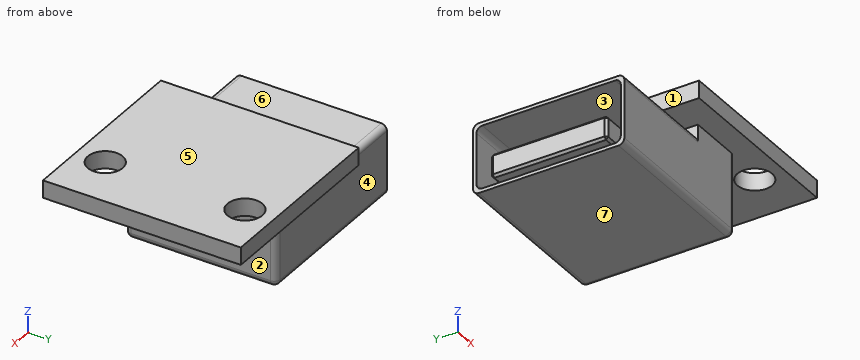
from build123d import *

# Parameters (mm, degrees)
SKETCH1_W           = 16
SKETCH1_H           = 17
BOSS_EXTRUDE1_DEPTH = 1.5
BOSS_EXTRUDE2_DEPTH = 6.5
SKETCH3_W           = 5.4
SKETCH3_H           = 12.4
SKETCH3_W_2         = 2
SKETCH3_H_2         = 10
CUT_EXTRUDE1_DEPTH  = 10
FILLET1_R           = 0.5
FILLET2_R           = 0.5
CHAMFER1_SIZE       = 0.2
SKETCH4_R           = 1.5
CUT_EXTRUDE2_DEPTH  = 10


with BuildPart() as part:
    # Sketch1 → Boss-Extrude1 (new body)
    with BuildSketch(Plane.XY):
        Rectangle(SKETCH1_W, SKETCH1_H)
    extrude(amount=BOSS_EXTRUDE1_DEPTH)

    # Sketch2 → Boss-Extrude2 (add, symmetric)
    with BuildSketch(Plane(origin=(0, 0, 0), x_dir=(1, 0, 0), z_dir=(0, 1, 0))):
        Polygon((-5, 0), (-5, 1), (-15, 1), (-15, 7), (0, 7), (0, 0), align=None)
    extrude(amount=BOSS_EXTRUDE2_DEPTH, both=True)

    # Sketch3 → Cut-Extrude1 (cut)
    with BuildSketch(Plane.ZY.offset(15)):
        with Locations((-4, 0)):
            Rectangle(SKETCH3_W, SKETCH3_H)
        with Locations((-5, 0)):
            Rectangle(SKETCH3_W_2, SKETCH3_H_2, mode=Mode.SUBTRACT)
    extrude(amount=-CUT_EXTRUDE1_DEPTH, mode=Mode.SUBTRACT)

    # Fillet1
    fillet1_edges = [part.edges().sort_by_distance(p)[0] for p in [
        (-7.5, -6.5, -7),
        (-10, -6.5, -1),
        (-7.5, 6.5, -7),
        (-10, 6.5, -1),
        (-10, 6.2, -6.7),
        (-10, 6.2, -1.3),
        (-10, -6.2, -1.3),
        (-10, -6.2, -6.7),
    ]]
    fillet(fillet1_edges, radius=FILLET1_R)

    # Fillet2
    fillet2_edges = [part.edges().sort_by_distance(p)[0] for p in [
        (0, -6.5, -3.25),
        (0, 6.5, -3.25),
        (0, 0, -7),
        (0, 6.353553391, -6.853553391),
        (0, -6.353553391, -6.853553391),
    ]]
    fillet(fillet2_edges, radius=FILLET2_R)

    # Chamfer1
    chamfer1_edges = [part.edges().sort_by_distance(p)[0] for p in [
        (-15, 0, -4),
        (-10, -5, -4),
        (-15, -5, -5),
        (-10, -5, -6),
        (-15, 0, -6),
        (-10, 5, -6),
        (-15, 5, -5),
        (-10, 5, -4),
    ]]
    chamfer(chamfer1_edges, length=CHAMFER1_SIZE)

    # Sketch4 → Cut-Extrude2 (cut)
    with BuildSketch(Plane(origin=(0, 0, 0), x_dir=(-1, 0, 0), z_dir=(0, 0, -1))):
        with Locations((-3.5, 6)):
            Circle(SKETCH4_R)
        with Locations((-3.5, -6)):
            Circle(SKETCH4_R)
    extrude(amount=-CUT_EXTRUDE2_DEPTH, mode=Mode.SUBTRACT)


solid = part.part
The listing builds one solid part. Answer for the finished solid, in the listing's coordinates (mm). Face numbers are marked on the shaded views. A direction names the side the tool comes from. Coordinates: 2 decimals unless noted, no trailing zeros. Write each loop counter-clockwise with the first axis right and the second up, starting at its lowest first coordinate (ties: lowest second). Pieces come first, ordered by that corner, then holes. Notation, with made-up numbers: (-40, 12) - (-19, 12) arc R21 cw to (-19, 22) - close; hole circle Ø10 at (58, 23.25). An arc over 180 degrees is marked (long way). Put each result on its own line as item: value.
1. Determine the mould class of the marked faces 4, 5, 6 and 7 for opening direction Z: pulls with the +Z half, pulls with the -Z half, needs draft (parallel to the pull), parting line crosses it, or undercut.
Answer sheet:
face 4: needs draft
face 5: pulls with the +Z half
face 6: undercut
face 7: pulls with the -Z half
2. A tool of negligible diameter and unlimited length cuts with its end or side. For the marked faces 1, 2 and 3, from which of +Z, -Z, +X, -X, +Y, -Y can it reach the whole face along a straight path? Write none if from no direction.
Answer sheet:
face 1: +Z, -X, +Y, -Y
face 2: -Z, +X, +Y, -Y
face 3: -X
3. Find the intervals of material crossed by line 1 along Y through (x, z) = (-13.5, -4.5); line 2 along Y through (x, z) = (3.5, 1); line 3 along Z through (x, y) = (-7, 5.75), in increasing order. Write a range as from..to.
Answer sheet:
line 1: y = -6.5..-6.2, -5..5, 6.2..6.5
line 2: y = -8.5..-7.5, -4.5..4.5, 7.5..8.5
line 3: z = -7..-6.7, -1.3..-1, 0..1.5
4. The part is cut by section B-B on x = 3.5. Give the vertices of the cut face in (y, z), plus the area to 3 significant figures.
Answer sheet:
outline: (-8.5, 0) - (-7.5, 0) - (-7.5, 1.5) - (-8.5, 1.5) - close; (-4.5, 0) - (4.5, 0) - (4.5, 1.5) - (-4.5, 1.5) - close; (7.5, 0) - (8.5, 0) - (8.5, 1.5) - (7.5, 1.5) - close
area: 16.5 mm^2
5. Flat-ended cylindrical pins translate along their axes: pin 1 Ø5 at (x, z) = (-12.5, -4) entering from -Y; pin 2 Ø1.6 at (y, z) = (2.5, 1) entering from -X; pin 3 Ø3.5 at (x, y) = (3.5, -6) entering from +Z; pin 4 Ø2 at (x, z) = (-11.5, -4.5) entering from +Y. Find the tip coordinate at first contact, or state that the pin passes through.
Answer sheet:
pin 1: stops at y = -6.5
pin 2: stops at x = -8
pin 3: stops at z = 1.5
pin 4: stops at y = 6.5
6. The part is cut by section D-D on y = 7. Give the vertices of the cut face in (x, z), plus the area to 3 significant figures.
Answer sheet:
outline: (-8, 0) - (2.38, 0) - (2.38, 1.5) - (-8, 1.5) - close; (4.62, 0) - (8, 0) - (8, 1.5) - (4.62, 1.5) - close
area: 20.6 mm^2
7. The part is cut by section C-C on z = 1. Give the vertices of the cut face in (x, y).
Answer sheet:
outline: (-8, -8.5) - (8, -8.5) - (8, 8.5) - (-8, 8.5) - close; hole circle Ø3 at (3.5, -6); hole circle Ø3 at (3.5, 6)
8. The part is cut by section A-A on x = -12. Give the vertices of the cut face in (y, z), plus the area to 3 significant figures.
Answer sheet:
outline: (-6.5, -6.5) arc R0.5 ccw to (-6, -7) - (6, -7) arc R0.5 ccw to (6.5, -6.5) - (6.5, -1.5) arc R0.5 ccw to (6, -1) - (-6, -1) arc R0.5 ccw to (-6.5, -1.5) - close; (-5, -5.8) - (-4.8, -6) - (4.8, -6) - (5, -5.8) - (5, -4.2) - (4.8, -4) - (-4.8, -4) - (-5, -4.2) - close; hole (-6.2, -6.2) arc R0.5 ccw to (-5.7, -6.7) - (5.7, -6.7) arc R0.5 ccw to (6.2, -6.2) - (6.2, -1.8) arc R0.5 ccw to (5.7, -1.3) - (-5.7, -1.3) arc R0.5 ccw to (-6.2, -1.8) - close
area: 31.0 mm^2
